from build123d import *

# Parameters (mm, degrees)
F0_W     = 158
F0_H     = 36
F0_R     = 2.5
F1_DEPTH = 6
F2_SIZE  = 0.5


with BuildPart() as f1:
    # F0 (on Top) → F1 (new body)
    with BuildSketch(Plane.XY):
        Rectangle(F0_W, F0_H)
        with Locations((-70, -9)):
            Circle(F0_R, mode=Mode.SUBTRACT)
        with Locations((0, -9)):
            Circle(F0_R, mode=Mode.SUBTRACT)
        with Locations((70, -9)):
            Circle(F0_R, mode=Mode.SUBTRACT)
        with Locations((-70, 9)):
            Circle(F0_R, mode=Mode.SUBTRACT)
        with Locations((0, 9)):
            Circle(F0_R, mode=Mode.SUBTRACT)
        with Locations((70, 9)):
            Circle(F0_R, mode=Mode.SUBTRACT)
    extrude(amount=F1_DEPTH)

    # F2
    f2_edges = [f1.edges().sort_by_distance(p)[0] for p in [
        (-67.5, -9, 3),
        (-72.5, -9, 0),
        (-72.5, -9, 6),
        (-67.5, 9, 3),
        (-72.5, 9, 0),
        (-72.5, 9, 6),
        (2.5, -9, 3),
        (-2.5, -9, 0),
        (-2.5, -9, 6),
        (2.5, 9, 3),
        (-2.5, 9, 0),
        (-2.5, 9, 6),
        (72.5, -9, 3),
        (67.5, -9, 0),
        (67.5, -9, 6),
        (72.5, 9, 3),
        (67.5, 9, 0),
        (67.5, 9, 6),
    ]]
    chamfer(f2_edges, length=F2_SIZE)


solid = f1.part
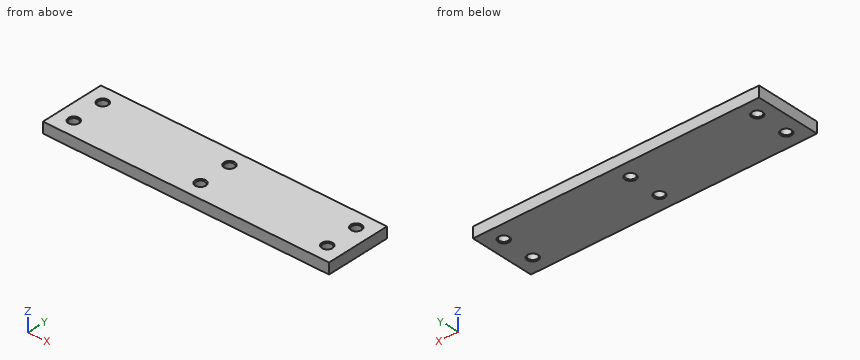
Verification items for the finished model (mm, model axes). Coordinates: 2 decimals unless noted, no trailing zeros. Order: outer loops, then holes, each group sorted by start corner. A loop starts at its lowest first (then second) coordinate and runs counter-clockwise, first axis right, second up. Notation, with made-up numbers: M 14,-4 L 19,-4 A25 cw 19,27 Z; hole C 23,51 d1. An arc over 180 degrees is marked long. One line per item, written item: value. Start each with the question number.
Item 1: Sectioned sample at C-C (x = 0). Enter the section's corners in (y, z).
Item 2: Sectioned sample at A-A (y = 9). Enter the section's corners in (x, z), then the cut area to 4 significant figures.
Item 3: Scan lines: probe 1 along Y at (x, z) = (-70, 2.7); probe 2 along Y at (x, z) = (69, 0.75); probe 3 along X at (y, z) = (11, 1.05). Record each from-to range of solid material in increasing order.
Item 4: Sectioned sample at B-B (z = 4.5). Enter the section's corners in (x, y).
Item 5: Gauge pin test, flat end, axial feed: pin 1 (6 mm diameter, centred on x = 49, y = 7, fed in from -Z). Record the tip position at first contact, or that the pin passes through.
Conclusion:
1. outline: M -18,0 L -12,0 L -11.5,0.5 L -11.5,5.5 L -12,6 L -18,6 Z; M -6.5,0.5 L -6,0 L 6,0 L 6.5,0.5 L 6.5,5.5 L 6,6 L -6,6 L -6.5,5.5 Z; M 11.5,0.5 L 12,0 L 18,0 L 18,6 L 12,6 L 11.5,5.5 Z
2. outline: M -79,0 L -73,0 L -72.5,0.5 L -72.5,5.5 L -73,6 L -79,6 Z; M -67.5,0.5 L -67,0 L -3,0 L -2.5,0.5 L -2.5,5.5 L -3,6 L -67,6 L -67.5,5.5 Z; M 2.5,0.5 L 3,0 L 67,0 L 67.5,0.5 L 67.5,5.5 L 67,6 L 3,6 L 2.5,5.5 Z; M 72.5,0.5 L 73,0 L 79,0 L 79,6 L 73,6 L 72.5,5.5 Z
2. area: 856.5 mm^2
3. probe 1: y = -18 to -11.5, -6.5 to 6.5, 11.5 to 18
3. probe 2: y = -18 to -11.29, -6.71 to 6.71, 11.29 to 18
3. probe 3: x = -79 to -71.5, -68.5 to -1.5, 1.5 to 68.5, 71.5 to 79
4. outline: M -79,-18 L 79,-18 L 79,18 L -79,18 Z; hole C -70,-9 d5; hole C -70,9 d5; hole C 0,-9 d5; hole C 0,9 d5; hole C 70,-9 d5; hole C 70,9 d5
5. pin 1: stops at z = 0
